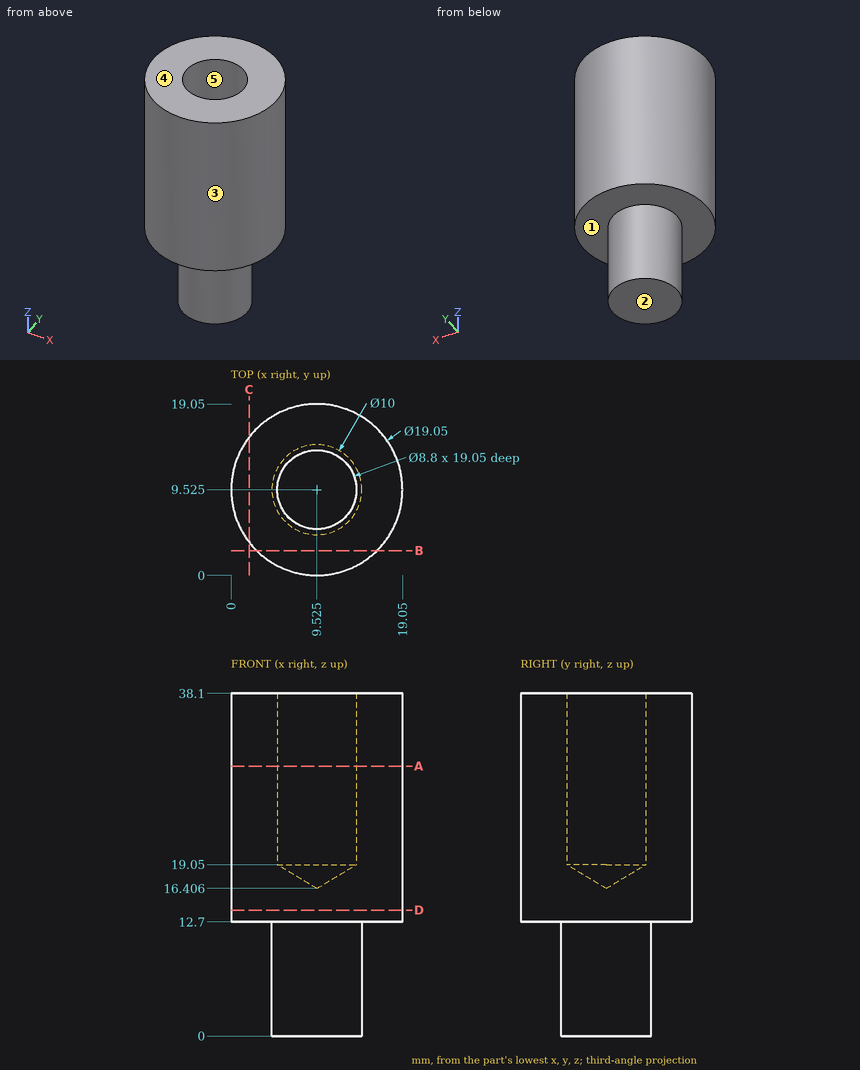
The drawing under review shows one solid part. Ordinate dimensions are in mm from its lowest x, y, z. A direction names the side the tool comes from. Coordinates: 2 decimals unless noted, no trailing zeros. Write each loop counter-clockwise with the first axis right and the second up, starting at its lowest first coordinate (ties: lowest second). Pieces come first, ordered by that corner, then holes. Notation, with made-up numbers: (0, -11.5) - (28, -11.5) arc R26 ccw to (28, 2.5) - close; hole circle Ø1 at (-1.5, 85). An arc over 180 degrees is marked (long way). Put each result on its own line as item: value.
1. Wall thickness on probe 1 along Y at (x, z) = (9.25, 21); probe 2 along X at (y, z) = (13, 29) (1 decimal); probe 3 along Z at (x, y) = (15.25, 7.75): over which ranges is each line inside the solid? List them lowest first.
Values found:
probe 1: 0 to 5.13, 13.92 to 19.05
probe 2: 0.7 to 6.8, 12.2 to 18.4
probe 3: 12.7 to 38.1
2. Add section C-C, the plane x = 2. Give the boundary of the cut face in (y, z), then the cut area to 3 significant figures.
Values found:
outline: (3.69, 12.7) - (15.36, 12.7) - (15.36, 38.1) - (3.69, 38.1) - close
area: 297 mm²
3. Mouldability with a two-part tool opening along Y and no side actions: class the marked faces 3, 4 and 5 as released by +Y, released by -Y, zero draft, split by the parting line, or undercut.
Values found:
face 3: split by the parting line
face 4: zero draft
face 5: undercut
4. Add section A-A, the plane z = 30. Give the boundary of the cut face in (x, y) (3 decimals).
Values found:
outline: circle Ø19.05 at (9.525, 9.525); hole circle Ø8.8 at (9.525, 9.525)
5. Add section B-B, the plane y = 2.75. Give the boundary of the cut face in (x, z).
Values found:
outline: (2.83, 12.7) - (16.22, 12.7) - (16.22, 38.1) - (2.83, 38.1) - close
6. Add section D-D, the plane z = 14. Give the boundary of the cut face in (x, y) (3 decimals).
Values found:
outline: circle Ø19.05 at (9.525, 9.525)
7. For pin 1 (4 mm diameter, centred on y = 11, z = 5.5, fed in from +X) (3 decimals); pin 2 (2 mm diameter, centred on y = 12.5, z = 19, fed in from -X); pin 3 (8 mm diameter, centred on x = 14.5, z = 11.5, fed in from -Y), all flat-tipped, find the tip position at first contact; note any pin that passes through.
Values found:
pin 1: x = 14.525
pin 2: x = 0.21
pin 3: y = 0.07
8. Machinability: for the marked faces 1 and 2, which of the approach directions +Z, -Z, +X, -X, +Y, -Y give a long, thin tool a straight path to every point of the face, cutting with its end or side? Answer none if there is none.
Values found:
face 1: -Z
face 2: -Z, +X, -X, +Y, -Y
